Source: three-view drawing plus pictorial views. Frame: mm from the lowest corner of the part. A direction names the side the tool comes from. Give positions to 0.01 mm unless a question says otherwise; leave off trailing zeros. Order: outer loops, then holes, each group sorted by start corner. A loop starts at its lowest first (then second) coordinate and runs counter-clockwise, first axis right, second up. Notation, with made-up numbers: (-32.75, -29.75) -> (-2.75, -29.75) arc R30 cw to (-2.75, -3.75) -> close; hole circle Ø6 at (13, 75). An arc over 180 degrees is marked (long way). Answer in a Markdown table with one row per item.
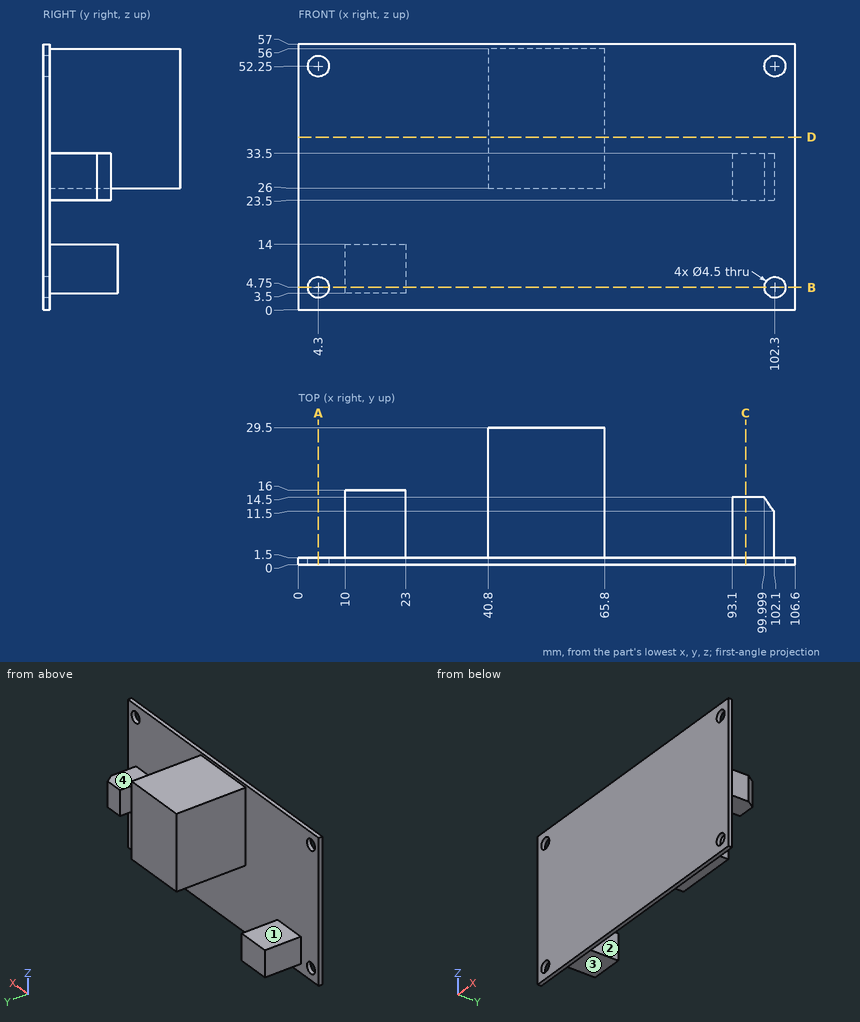
(1) Section query D-D (z = 37). Return the cut outline in (x, y), plus the area to 3 significant figures.
A:
| item | result |
|---|---|
| outline | (0, 0) -> (106.6, 0) -> (106.6, 1.5) -> (65.8, 1.5) -> (65.8, 29.5) -> (40.8, 29.5) -> (40.8, 1.5) -> (0, 1.5) -> close |
| area | 860 mm^2 |
(2) Access query for the marked faces 1, 2, 3 and 4. Directions: +Z, -Z, +X, -X, +Y, -Y. A direction counts if a zero-diameter tool reaches every point of the face in a straight line with its end or side. Return the directions, or none.
A:
| item | result |
|---|---|
| face 1 | +Z, +X, -X, +Y |
| face 2 | +Z, -Z, +X, +Y |
| face 3 | -Z, +X, -X, +Y |
| face 4 | +Z, +X, +Y |
(3) Ray query, probe 1 along Z at (x, y) = (102.3, 0.45); probe 2 along X at (y, z) = (6, 30.5); probe 3 along Z at (x, y) = (43.5, 10). Return the intervals inside material, ascending.
A:
| item | result |
|---|---|
| probe 1 | z = 0 to 2.5, 7 to 50, 54.5 to 57 |
| probe 2 | x = 40.8 to 65.8, 93.1 to 102.1 |
| probe 3 | z = 26 to 56 |
(4) Section query B-B (z = 4.75). Return the cut outline in (x, y).
A:
| item | result |
|---|---|
| outline | (0, 0) -> (2.05, 0) -> (2.05, 1.5) -> (0, 1.5) -> close; (6.55, 0) -> (100.05, 0) -> (100.05, 1.5) -> (23, 1.5) -> (23, 16) -> (10, 16) -> (10, 1.5) -> (6.55, 1.5) -> close; (104.55, 0) -> (106.6, 0) -> (106.6, 1.5) -> (104.55, 1.5) -> close |
(5) Section query A-A (x = 4.3). Return the cut outline in (y, z).
A:
| item | result |
|---|---|
| outline | (0, 0) -> (1.5, 0) -> (1.5, 2.5) -> (0, 2.5) -> close; (0, 7) -> (1.5, 7) -> (1.5, 50) -> (0, 50) -> close; (0, 54.5) -> (1.5, 54.5) -> (1.5, 57) -> (0, 57) -> close |
(6) First-contact query: pin 1 Ø4 at (x, z) = (32, 17) entering from +Y; pin 2 Ø3 at (y, z) = (4.5, 27) entering from +X; pin 3 Ø11.5 at (y, z) = (12, 8.5) entering from +X. Flat tips, straight axial feed; report the tip coordinate or a pass-through.
A:
| item | result |
|---|---|
| pin 1 | stops at y = 1.5 |
| pin 2 | stops at x = 102.1 |
| pin 3 | stops at x = 23 |
(7) Section query C-C (x = 96). Return the cut outline in (y, z).
A:
| item | result |
|---|---|
| outline | (0, 0) -> (1.5, 0) -> (1.5, 23.5) -> (14.5, 23.5) -> (14.5, 33.5) -> (1.5, 33.5) -> (1.5, 57) -> (0, 57) -> close |
